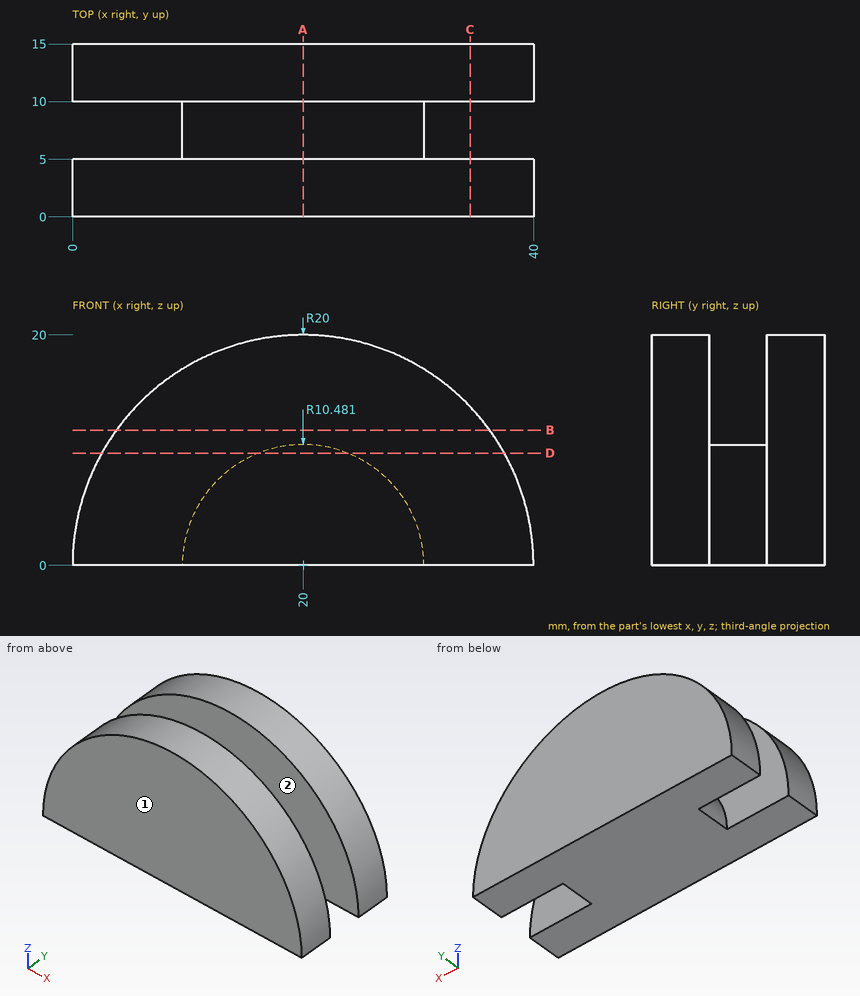
The drawing under review shows one solid part. Ordinate dimensions are in mm from its lowest x, y, z. A direction names the side the tool comes from. Round coordinates to 2 decimals unless told otherwise and drop trailing zeros. Loops run counter-clockwise (first coordinate to the right, second up) from the corner with the lowest first, then second, coordinate; pieces in that order, holes last. Notation, with made-up numbers: (-21.5, 34) -> (7.5, 34) arc R22 ccw to (7.5, 55) -> close; hole circle Ø4 at (49, 35.25). An arc over 180 degrees is marked (long way). Answer in a Markdown table with one row per item.
1) Consider section D-D, the plane z = 9.75. Write out the cut boundary in (x, y) (1 decimal).
Taken from the geometry:
| item | result |
|---|---|
| outline | (2.5, 0) -> (37.5, 0) -> (37.5, 5) -> (23.8, 5) -> (23.8, 10) -> (37.5, 10) -> (37.5, 15) -> (2.5, 15) -> (2.5, 10) -> (16.2, 10) -> (16.2, 5) -> (2.5, 5) -> close |
2) Consider section B-B, the plane z = 11.75. Write out the cut boundary in (x, y) (1 decimal), plus the area to 3 significant figures.
Taken from the geometry:
| item | result |
|---|---|
| outline | (3.8, 0) -> (36.2, 0) -> (36.2, 5) -> (3.8, 5) -> close; (3.8, 10) -> (36.2, 10) -> (36.2, 15) -> (3.8, 15) -> close |
| area | 324 mm² |
3) Tool access review of the marked faces 1 and 2: name each direction out of +Z, -Z, +X, -X, +Y, -Y from which nothing blocks a thin tool from reaching the whole face with its end or side.
Taken from the geometry:
| item | result |
|---|---|
| face 1 | +Z, -Z, +X, -X, -Y |
| face 2 | +Z |
4) Consider section A-A, the plane x = 20. Write out the cut boundary in (y, z), plus the area to 3 significant figures.
Taken from the geometry:
| item | result |
|---|---|
| outline | (0, 0) -> (15, 0) -> (15, 20) -> (10, 20) -> (10, 10.48) -> (5, 10.48) -> (5, 20) -> (0, 20) -> close |
| area | 252 mm² |
5) For pin 1 Ø1.5 at (x, z) = (22, 8.5) entering from -Y; pin 2 Ø6 at (y, z) = (12, 11) entering from +X; pin 3 Ø4 at (y, z) = (7.5, 9.5) entering from -X, all flat-tipped, find the tip position at first contact; note any pin that passes through.
Taken from the geometry:
| item | result |
|---|---|
| pin 1 | stops at y = 0 |
| pin 2 | stops at x = 38.33 |
| pin 3 | stops at x = 12.68 |
6) Consider section C-C, the plane x = 34.5. Write out the cut boundary in (y, z) (1 decimal).
Taken from the geometry:
| item | result |
|---|---|
| outline | (0, 0) -> (5, 0) -> (5, 13.8) -> (0, 13.8) -> close; (10, 0) -> (15, 0) -> (15, 13.8) -> (10, 13.8) -> close |
7) Wall thickness on line 1 along Y through (x, z) = (33.5, 10.75); line 2 along Z through (x, y) = (20, 11.5); line 3 along Z through (x, y) = (11.5, 2.5) (1 decimal): over which ranges is each line inside the solid? List them lowest first.
Taken from the geometry:
| item | result |
|---|---|
| line 1 | y = 0 to 5, 10 to 15 |
| line 2 | z = 0 to 20 |
| line 3 | z = 0 to 18.1 |
